from build123d import *

# Parameters (mm, degrees)
F2_R     = 81
F3_DEPTH = 5
F4_R     = 1
F5_W     = 8
F5_H     = 12
F5_R     = 2.5
F7_DEPTH = 12.5
F6_W     = 8
F6_H     = 12
F6_R     = 1.75
F8_DEPTH = 12.5


with BuildPart() as f1:
    # F0 (on Front) → F1 (revolve)
    with BuildSketch(Plane.XZ):
        with BuildLine():
            Line((-85, -3), (-77, -3))
            Line((-77, -3), (-77, 0))
            Line((-77, 0), (-77, 7))
            Line((-77, 7), (-88.5, 7))
            Line((-88.5, 7), (-88.5, 1))
            ThreePointArc((-88.5, 1), (-87.380683, -1.907671), (-87, -5))
            Line((-87, -5), (-87, -11))
            Line((-87, -11), (-85, -11))
            Line((-85, -11), (-85, -3))
        make_face()
    revolve(axis=Axis((0, 0, -0.2651), (0, 0, 1)))

    # F2 (on Top) → F3 (cut)
    with BuildSketch(Plane.XY):
        Circle(F2_R)
    extrude(amount=F3_DEPTH, mode=Mode.SUBTRACT)

    # F4
    f4_edges = [f1.edges().sort_by_distance(p)[0] for p in [
        (87, 0, -11),
    ]]
    fillet(f4_edges, radius=F4_R)

    # F5 (on Front) → F7 (join, symmetric)
    with BuildSketch(Plane.XZ):
        with Locations((-89.5, -2)):
            Rectangle(F5_W, F5_H)
        with Locations((-89, -2)):
            Circle(F5_R, mode=Mode.SUBTRACT)
    extrude(amount=F7_DEPTH, both=True)

    # F6 (on Front) → F8 (join, symmetric)
    with BuildSketch(Plane.XZ):
        with Locations((89.5, -2)):
            Rectangle(F6_W, F6_H)
        with Locations((89, -2)):
            Circle(F6_R, mode=Mode.SUBTRACT)
    extrude(amount=F8_DEPTH, both=True)


solid = f1.part
Build history of the part. All positions in model axes, mm. A direction names the side the tool comes from. Coordinates: 2 decimals unless noted, no trailing zeros. One line per item, written item: value.
(1) Mould opens along Z. For faces 5 (the flat face through (72, -30, 5)), 6 (the flat face through (93.5, 0, -2)), 7 (the flat face through (-66, -40, 7)), 8 (the flat face through (20, -83, -11)) say: pulls with the +Z half, pulls with the -Z half, needs draft (parallel to the pull), parting line crosses it, or undercut.
Checked values:
face 5: undercut
face 6: needs draft
face 7: pulls with the +Z half
face 8: pulls with the -Z half
(2) Tool access for faces 1 (the flat face through (72, -30, 0)), 2 (the cylindrical face through (67.453, 51.721, -6.944)), 3 (the flat face through (91, -12.5, -3)), 4 (the flat face through (-91.5, -12.5, -3.2)): list every direction of +Z, -Z, +X, -X, +Y, -Y with a clear straight run to the whole face (end or side of a thin tool).
Checked values:
face 1: none
face 2: -Z
face 3: -Z, +X, -Y
face 4: -Z, -X, -Y
(3) Probe line 1 (Y direction, x = 0, z = 2.6); line 2 (Y direction, x = 0, z = 6.2); line 3 (X direction, y = -10, z = -4). List the from-to ranges inside material, lowest first. Write a range as [from, to].
Checked values:
line 1: [-88.5, -81], [81, 88.5]
line 2: [-88.5, -77], [77, 88.5]
line 3: [-93.5, -90.5], [-87.5, -84.41], [84.41, 93.5]
(4) Drop flat-ended pins along their axis: pin 1 Ø3 at (x, y) = (70.5, -38) entering from -Z; pin 2 Ø3 at (y, z) = (-33, 2.5) entering from -X; pin 3 Ø3 at (x, y) = (-90.5, 3.5) entering from +Z; pin 4 Ø2 at (x, z) = (88.5, -2.5) entering from +Y. Give the stop position or say it passes through.
Checked values:
pin 1: z = -3
pin 2: x = -82.7
pin 3: z = 4
pin 4: through
(5) Slice it at A-A, the plane y = -9. Count the separate pieces of the cut face and the enclosed holes in it, plus the area to 3 significant figures.
Checked values:
separate pieces: 2
enclosed holes: 2
area: 341 mm2
